Build history of the part. All positions in model axes, mm. A direction names the side the tool comes from. Give positions to 0.01 mm unless a question says otherwise; leave off trailing zeros. Write each loop counter-clockwise with the first axis right and the second up, starting at its lowest first coordinate (ties: lowest second). Pieces come first, ordered by that corner, then holes.
from build123d import *

# Parameters (mm, degrees)
SKETCH1_W           = 53
SKETCH1_H           = 20.877946607
SKETCH1_R           = 2.5
SKETCH1_R_2         = 2
BOSS_EXTRUDE1_DEPTH = 4


with BuildPart() as part:
    # Sketch1 → Boss-Extrude1 (new body)
    with BuildSketch(Plane.XY):
        Polygon((-70, 27.877946607), (-70, -7), (70, -7), (70, 27.877946607), (105.826370741, 27.877946607), (105.826370741, 41.877946607), (-105.826370741, 41.877946607), (-105.826370741, 27.877946607), align=None)
        with Locations((33.5, 17.438973303)):
            Rectangle(SKETCH1_W, SKETCH1_H, mode=Mode.SUBTRACT)
        with Locations((0, 9)):
            Circle(SKETCH1_R, mode=Mode.SUBTRACT)
        with Locations((-33.5, 17.438973303)):
            Rectangle(SKETCH1_W, SKETCH1_H, mode=Mode.SUBTRACT)
        with Locations((60, 0)):
            Circle(SKETCH1_R, mode=Mode.SUBTRACT)
        with Locations((-60, 0)):
            Circle(SKETCH1_R, mode=Mode.SUBTRACT)
        with Locations((-30, 0)):
            Circle(SKETCH1_R_2, mode=Mode.SUBTRACT)
        Circle(SKETCH1_R, mode=Mode.SUBTRACT)
        with Locations((30, 0)):
            Circle(SKETCH1_R_2, mode=Mode.SUBTRACT)
        with Locations((-30, 34.877946607)):
            Circle(SKETCH1_R_2, mode=Mode.SUBTRACT)
        with Locations((-95.826370741, 34.877946607)):
            Circle(SKETCH1_R, mode=Mode.SUBTRACT)
        with Locations((0, 34.877946607)):
            Circle(SKETCH1_R, mode=Mode.SUBTRACT)
        with Locations((95.826370741, 34.877946607)):
            Circle(SKETCH1_R, mode=Mode.SUBTRACT)
        with Locations((30, 34.877946607)):
            Circle(SKETCH1_R_2, mode=Mode.SUBTRACT)
    extrude(amount=BOSS_EXTRUDE1_DEPTH)


solid = part.part
(1) Drop flat-ended pins along their axis: pin 1 (1 mm diameter, centred on y = 17.5, z = 0.5, fed in from +X); pin 2 (4.5 mm diameter, centred on x = -60, y = 0, fed in from +Z); pin 3 (2 mm diameter, centred on y = 14, z = 2.5, fed in from -X); pin 4 (2 mm diameter, centred on x = -89, z = 1.5, fed in from -Y). Give the stop position or say it passes through.
(2) Saw through at A-A, the plane x = 16. List the corners of the cut face in (y, z).
(3) 3-axis set-ups, long thin cutter, end or side, ignore diameter. For faces 1 (the face through (-34, 27.878, 2)), 2 (the face through (105.826, 35, 2)), 3 (the face through (70, 10, 2)): which of +Z, -Z, +X, -X, +Y, -Y reach the whole face in a straight line?
(4) Saw through at D-D, the plane y = 21.5. List the corners of the cut face in (x, z).
(5) Mould opens along Y. For faces 4 (the face through (-105.826, 35, 2)), 5 (the face through (31.908, 0.601, 1.972)), 6 (the face through (-88, 27.878, 2)) say: +Y half, -Y half, draft (parallel to the pull), parting line (faces both ways), or undercut.
(6) Saw through at C-C, the plane y = 9. List the corners of the cut face in (x, z).
(7) Saw through at B-B, the plane y = 0. List the corners of the cut face in (x, z), plus the area to 3 significant figures.
(8) Probe line 1 (X direction, y = 27, z = 1); line 2 (Y direction, x = -31, z = 0.5); line 3 (X direction, y = 5, z = 2.35). List the from-to ranges inside material, lowest first.
Computed values:
1. pin 1: stops at x = 70
1. pin 2: passes through
1. pin 3: stops at x = -70
1. pin 4: stops at y = 27.88
2. outline: (-7, 0) - (7, 0) - (7, 4) - (-7, 4) - close; (27.88, 0) - (41.88, 0) - (41.88, 4) - (27.88, 4) - close
3. face 1: +Z, -Z
3. face 2: +Z, -Z, +X, +Y, -Y
3. face 3: +Z, -Z, +X, -Y
4. outline: (-70, 0) - (-60, 0) - (-60, 4) - (-70, 4) - close; (-7, 0) - (7, 0) - (7, 4) - (-7, 4) - close; (60, 0) - (70, 0) - (70, 4) - (60, 4) - close
5. face 4: draft
5. face 5: undercut
5. face 6: -Y half
6. outline: (-70, 0) - (-60, 0) - (-60, 4) - (-70, 4) - close; (-7, 0) - (-2.5, 0) - (-2.5, 4) - (-7, 4) - close; (2.5, 0) - (7, 0) - (7, 4) - (2.5, 4) - close; (60, 0) - (70, 0) - (70, 4) - (60, 4) - close
7. outline: (-70, 0) - (-62.5, 0) - (-62.5, 4) - (-70, 4) - close; (-57.5, 0) - (-32, 0) - (-32, 4) - (-57.5, 4) - close; (-28, 0) - (-2.5, 0) - (-2.5, 4) - (-28, 4) - close; (2.5, 0) - (28, 0) - (28, 4) - (2.5, 4) - close; (32, 0) - (57.5, 0) - (57.5, 4) - (32, 4) - close; (62.5, 0) - (70, 0) - (70, 4) - (62.5, 4) - close
7. area: 468 mm2
8. line 1: x = -70 to -60, -7 to 7, 60 to 70
8. line 2: y = -7 to -1.73, 1.73 to 7, 27.88 to 33.15, 36.61 to 41.88
8. line 3: x = -70 to 70
